Part model, mm, in its own coordinate system. Round coordinates to 2 decimals unless told otherwise and drop trailing zeros. Write each loop counter-clockwise with the first axis right and the second up, starting at its lowest first coordinate (ties: lowest second). Pieces come first, ordered by that corner, then holes.
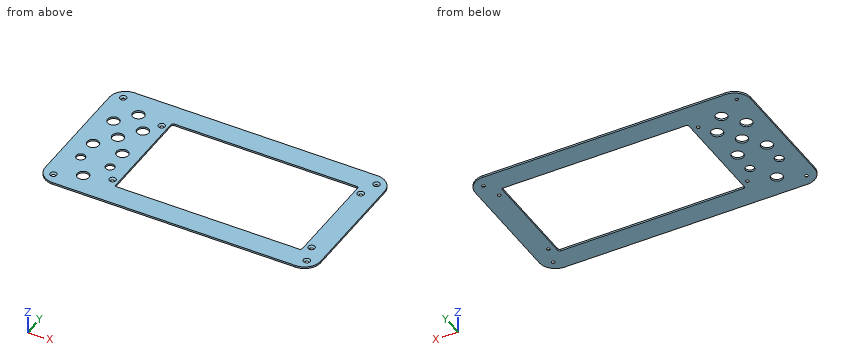
```python
from build123d import *

# Parameters (mm, degrees)
EXTRUDE1_DEPTH                                 = 1.25
CUT_EXTRUDE4_DEPTH                             = 3.5
ESBO_O6_R                                      = 8
ESBO_O6_R_2                                    = 6
CORTE_EXTRUS_O1_DEPTH                          = 10
ESBO_O7_R                                      = 1
CORTE_EXTRUS_O2_DEPTH                          = 3.5
ESCAREADO_PARA_PARAFUSO_ALLEN_SEXTAV_2_A_COUNT = 2
ESCAREADO_PARA_PARAFUSO_ALLEN_SEXTAV_2_A_PITCH = 120
ESCAREADO_PARA_PARAFUSO_ALLEN_SEXTAV_3_COUNT   = 2
ESCAREADO_PARA_PARAFUSO_ALLEN_SEXTAV_3_PITCH   = 296.379823875
ESCAREADO_PARA_PARAFUSO_ALLEN_SEXTAV_4_COUNT   = 2
ESCAREADO_PARA_PARAFUSO_ALLEN_SEXTAV_4_PITCH   = 271


with BuildPart() as part:
    # Sketch1 → Extrude1 (new body, symmetric)
    with BuildSketch(Plane.XY):
        with BuildLine():
            Line((-165.5, 100), (165.5, 100))
            ThreePointArc((165.5, 100), (181.056349186, 93.556349186), (187.5, 78))
            Line((187.5, 78), (187.5, -78))
            ThreePointArc((187.5, -78), (181.056349186, -93.556349186), (165.5, -100))
            Line((165.5, -100), (-165.5, -100))
            ThreePointArc((-165.5, -100), (-181.056349186, -93.556349186), (-187.5, -78))
            Line((-187.5, -78), (-187.5, 78))
            ThreePointArc((-187.5, 78), (-181.056349186, 93.556349186), (-165.5, 100))
        make_face()
    extrude(amount=EXTRUDE1_DEPTH, both=True)

    # Sketch5 → Cut-Extrude4 (cut, through all)
    with BuildSketch(Plane.XY.offset(1.25)):
        with BuildLine():
            Line((-95, 70), (154, 70))
            ThreePointArc((154, 70), (155.767766953, 69.267766953), (156.5, 67.5))
            Line((156.5, 67.5), (156.5, -67.5))
            ThreePointArc((156.5, -67.5), (155.767766953, -69.267766953), (154, -70))
            Line((154, -70), (-95, -70))
            ThreePointArc((-95, -70), (-96.767766953, -69.267766953), (-97.5, -67.5))
            Line((-97.5, -67.5), (-97.5, 67.5))
            ThreePointArc((-97.5, 67.5), (-96.767766953, 69.267766953), (-95, 70))
        make_face()
    extrude(amount=-CUT_EXTRUDE4_DEPTH, mode=Mode.SUBTRACT)

    # Esboço1 → Escareado para parafuso Allen sextavado (revolve, cut)
    with BuildSketch(Plane(origin=(172.5, 85, 1.25), x_dir=(0, -1, 0), z_dir=(1, 0, 0))):
        Polygon((0, 0), (0, 2.5), (2.25, 2.5), (2.25, 2.23), (4.48, 0), align=None)
    escareado_para_parafuso_allen_sextavado = revolve(axis=Axis((172.5, 85, 7.6), (0, 0, -1)), mode=Mode.SUBTRACT)

    # Espelhar2: Escareado para parafuso Allen sextavado across plane
    add(escareado_para_parafuso_allen_sextavado.mirror(Plane(origin=(0, 0, 0), x_dir=(0, 0, 1), z_dir=(1, 0, 0))), mode=Mode.SUBTRACT)

    # Espelhar3: Escareado para parafuso Allen sextavado across plane
    add(escareado_para_parafuso_allen_sextavado.mirror(Plane.ZX), mode=Mode.SUBTRACT)

    # Espelhar3 copy 1 sketch → Espelhar3 copy 1 (revolve, cut)
    with BuildSketch(Plane(origin=(-172.5, -85, 1.25), x_dir=(0, 1, 0), z_dir=(-1, 0, 0))):
        Polygon((0, 0), (0, 2.5), (2.25, 2.5), (2.25, 2.23), (4.48, 0), align=None)
    revolve(axis=Axis((-172.5, -85, 7.6), (0, 0, -1)), mode=Mode.SUBTRACT)

    # Esboço6 → Corte-extrusão1 (cut)
    with BuildSketch(Plane.XY.offset(1.25)):
        with Locations((-140.5, 65)):
            Circle(ESBO_O6_R)
        with Locations((-120.5, 40)):
            Circle(ESBO_O6_R)
        with Locations((-160.5, 40)):
            Circle(ESBO_O6_R)
        with Locations((-140.5, 15)):
            Circle(ESBO_O6_R)
        with Locations((-120.5, -10)):
            Circle(ESBO_O6_R)
        with Locations((-160.5, -10)):
            Circle(ESBO_O6_R)
        with Locations((-140.5, -70)):
            Circle(ESBO_O6_R)
        with Locations((-120.5, -40)):
            Circle(ESBO_O6_R_2)
        with Locations((-160.5, -40)):
            Circle(ESBO_O6_R_2)
    extrude(amount=-CORTE_EXTRUS_O1_DEPTH, mode=Mode.SUBTRACT)

    # Esboço7 → Corte-extrusão2 (cut, through all)
    with BuildSketch(Plane.XY.offset(1.25)):
        with Locations((-106, -60)):
            Circle(ESBO_O7_R)
        with Locations((-106, 60)):
            Circle(ESBO_O7_R)
        with Locations((165, 60)):
            Circle(ESBO_O7_R)
        with Locations((165, -60)):
            Circle(ESBO_O7_R)
    extrude(amount=-CORTE_EXTRUS_O2_DEPTH, mode=Mode.SUBTRACT)

    # Esboço11 → Escareado para parafuso Allen sextav 2 (revolve, cut)
    with BuildSketch(Plane(origin=(-106, 60, 1.25), x_dir=(0, -1, 0), z_dir=(1, 0, 0))):
        Polygon((0, 0), (0, 2.5), (2.25, 2.5), (2.25, 2.23), (4.48, 0), align=None)
    escareado_para_parafuso_allen_sextav_2 = revolve(axis=Axis((-106, 60, 7.6), (0, 0, -1)), mode=Mode.SUBTRACT)

    # Escareado para parafuso Allen sextav 2 a: Escareado para parafuso Allen sextav 2 ×2
    with Locations(*[(0, -i * ESCAREADO_PARA_PARAFUSO_ALLEN_SEXTAV_2_A_PITCH, 0) for i in range(1, ESCAREADO_PARA_PARAFUSO_ALLEN_SEXTAV_2_A_COUNT)]):
        add(escareado_para_parafuso_allen_sextav_2, mode=Mode.SUBTRACT)

    # Escareado para parafuso Allen sextav 3: Escareado para parafuso Allen sextav 2 ×2
    with Locations(*[Vector(0.914367235, -0.40488586, 0) * (i * ESCAREADO_PARA_PARAFUSO_ALLEN_SEXTAV_3_PITCH) for i in range(1, ESCAREADO_PARA_PARAFUSO_ALLEN_SEXTAV_3_COUNT)]):
        add(escareado_para_parafuso_allen_sextav_2, mode=Mode.SUBTRACT)

    # Escareado para parafuso Allen sextav 4: Escareado para parafuso Allen sextav 2 ×2
    with Locations(*[(i * ESCAREADO_PARA_PARAFUSO_ALLEN_SEXTAV_4_PITCH, 0, 0) for i in range(1, ESCAREADO_PARA_PARAFUSO_ALLEN_SEXTAV_4_COUNT)]):
        add(escareado_para_parafuso_allen_sextav_2, mode=Mode.SUBTRACT)


solid = part.part
```
Q1. Cut at D-D on y = 15. Write the cut outline in (x, z), plus the area to 4 significant figures.
Values follow:
outline: (-187.5, -1.25) - (-148.5, -1.25) - (-148.5, 1.25) - (-187.5, 1.25) - close; (-132.5, -1.25) - (-97.5, -1.25) - (-97.5, 1.25) - (-132.5, 1.25) - close; (156.5, -1.25) - (187.5, -1.25) - (187.5, 1.25) - (156.5, 1.25) - close
area: 262.5 mm2
Q2. Cut at A-A on y = -40. Write the cut outline in (x, z).
Values follow:
outline: (-187.5, -1.25) - (-166.5, -1.25) - (-166.5, 1.25) - (-187.5, 1.25) - close; (-154.5, -1.25) - (-126.5, -1.25) - (-126.5, 1.25) - (-154.5, 1.25) - close; (-114.5, -1.25) - (-97.5, -1.25) - (-97.5, 1.25) - (-114.5, 1.25) - close; (156.5, -1.25) - (187.5, -1.25) - (187.5, 1.25) - (156.5, 1.25) - close
Q3. Drop flat-ended pins along their axis: pin 1 (9.5 mm diameter, centred on x = -140.5, y = 65, fed in from -Z); pin 2 (6 mm diameter, centred on x = 172.5, y = -85, fed in from +Z); pin 3 (7 mm diameter, centred on x = -106, y = 60, fed in from +Z). Give the stop position or say it passes through.
Values follow:
pin 1: passes through
pin 2: stops at z = -0.23
pin 3: stops at z = 0.27
Q4. Cut at C-C on x = 146.5. Write the cut outline in (y, z).
Values follow:
outline: (-100, -1.25) - (-70, -1.25) - (-70, 1.25) - (-100, 1.25) - close; (70, -1.25) - (100, -1.25) - (100, 1.25) - (70, 1.25) - close
Q5. Wall check: L1, parallel to Y at x = -140.5, z = 0.55; L2, parallel to Y at x = -160.5, z = -0.45; L3, parallel to X at y = 59.5, z = 0.7. Give the ranges that are in metal, low to high.
Values follow:
L1: y = -100 to -78, -62 to 7, 23 to 57, 73 to 100
L2: y = -100 to -46, -34 to -18, -2 to 32, 48 to 100
L3: x = -187.5 to -146.31, -134.69 to -109.9, -102.1 to -97.5, 156.5 to 161.1, 168.9 to 187.5
Q6. Cut at B-B on z = -0.1. State how many separate pieces and enclosed holes the cut face has, plus the area to 4 significant figures.
Values follow:
separate pieces: 1
enclosed holes: 18
area: 37,150 mm2
